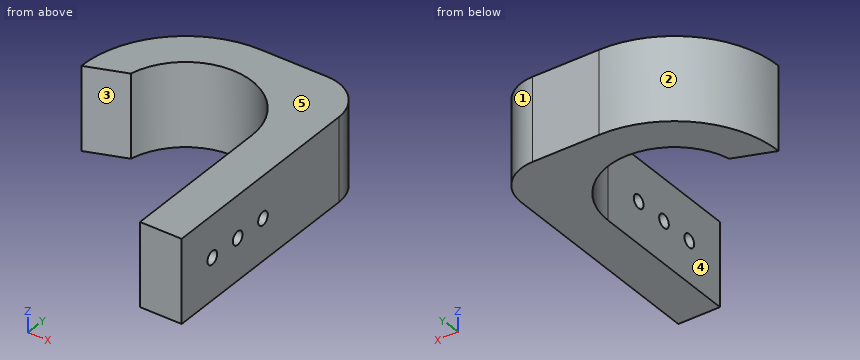
from build123d import *

# Parameters (mm, degrees)
F1_DEPTH = 25.4
F2_R     = 2.032
F3_DEPTH = 12.7


with BuildPart() as f1:
    # F0 (on Top) → F1 (new body)
    with BuildSketch(Plane.XY):
        with BuildLine():
            ThreePointArc((-19.8374, 4.402268), (2.214321, 20.19899), (20.32, 0))
            Line((20.32, 0), (20.32, -47.217399))
            Line((20.32, -47.217399), (33.02, -47.217399))
            Line((33.02, -47.217399), (33.02, 19.05))
            ThreePointArc((33.02, 19.05), (29.300256, 28.030256), (20.32, 31.75))
            Line((20.32, 31.75), (0, 31.75))
            ThreePointArc((0, 31.75), (-22.45064, 22.45064), (-31.75, 0))
            Line((-31.75, 0), (-19.8374, 4.402268))
        make_face()
    extrude(amount=F1_DEPTH)

    # F2 (on face) → F3 (cut, through all)
    with BuildSketch(Plane.YZ.offset(33.02)):
        with Locations((-34.291968, 12.7)):
            Circle(F2_R)
        with Locations((-23.623968, 12.7)):
            Circle(F2_R)
        with Locations((-12.955968, 12.7)):
            Circle(F2_R)
    extrude(amount=-F3_DEPTH, mode=Mode.SUBTRACT)


solid = f1.part
Input: part model. Units: mm. Frame: model coordinates. Face numbers are marked on the shaded views. A direction names the side the tool comes from. Give positions to 0.01 mm unless a question says otherwise; leave off trailing zeros. Order: outer loops, then holes, each group sorted by start corner. A loop starts at its lowest first (then second) coordinate and runs counter-clockwise, first axis right, second up.
Q1. Section D-D on y = -27. Output: boundary loops of the cut face in (x, z), and give its area (3 significant figures).
Checked values:
outline: (20.32, 0) - (33.02, 0) - (33.02, 25.4) - (20.32, 25.4) - close
area: 323 mm2
Q2. Contact query for a flat-ended pin moving along its axis: pin 1 Ø6 at (y, z) = (-36.5, 20) entering from -X. Output: stop coordinate, or through.
Checked values:
pin 1: stops at x = 20.32
Q3. Section A-A on z = 12.7. Output: boundary loops of the cut face in (x, y).
Checked values:
outline: (-31.75, 0) - (-19.84, 4.4) arc R20.32 cw to (20.32, 0) - (20.32, -10.92) - (33.02, -10.92) - (33.02, 19.05) arc R12.7 ccw to (20.32, 31.75) - (0, 31.75) arc R31.75 ccw to start; (20.32, -47.22) - (33.02, -47.22) - (33.02, -36.32) - (20.32, -36.32) - close; (20.32, -32.26) - (33.02, -32.26) - (33.02, -25.66) - (20.32, -25.66) - close; (20.32, -21.59) - (33.02, -21.59) - (33.02, -14.99) - (20.32, -14.99) - close
Q4. Draft query along X for the marked faces 1, 2 and 3. Return one class per face: +X half, -X half, draft (parallel to the pull), parting line (faces both ways), or undercut.
Checked values:
face 1: +X half
face 2: -X half
face 3: undercut
Q5. Set-up query: the marked faces 4 and 5. Return all of +Z, -Z, +X, -X, +Y, -Y with unobstructed straight access to the full face (end or side cutting, diameter ignored); none if empty.
Checked values:
face 4: +Z, -Z, -X, -Y
face 5: +Z, +X, -X, +Y, -Y
Q6. Section C-C on x = 26. Output: boundary loops of the cut face in (y, z).
Checked values:
outline: (-47.22, 0) - (30.41, 0) - (30.41, 25.4) - (-47.22, 25.4) - close; hole circle Ø4.06 at (-34.29, 12.7); hole circle Ø4.06 at (-23.62, 12.7); hole circle Ø4.06 at (-12.96, 12.7)
Q7. Section B-B on z = 23.5. Output: boundary loops of the cut face in (x, y).
Checked values:
outline: (-31.75, 0) - (-19.84, 4.4) arc R20.32 cw to (20.32, 0) - (20.32, -47.22) - (33.02, -47.22) - (33.02, 19.05) arc R12.7 ccw to (20.32, 31.75) - (0, 31.75) arc R31.75 ccw to start
Q8. Ray query, probe 1 along X at (y, z) = (-31, 18); probe 2 along X at (y, z) = (14.5, 16.25); probe 3 along X at (y, z) = (11, 14). Return the intervals inside material, ascending.
Checked values:
probe 1: x = 20.32 to 33.02
probe 2: x = -28.25 to -14.24, 14.24 to 33.02
probe 3: x = -29.78 to -17.09, 17.09 to 33.02
